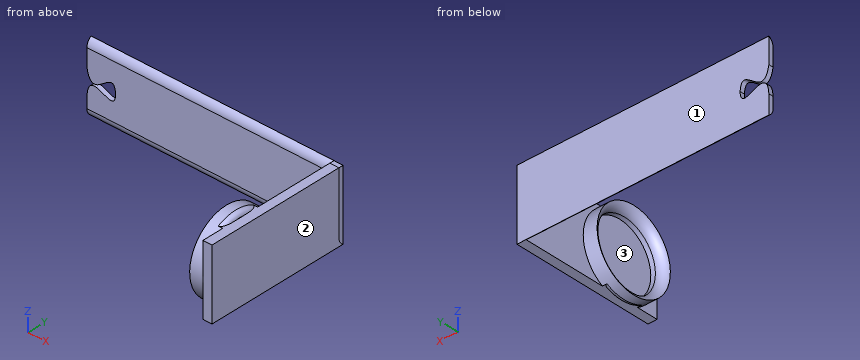
```python
from build123d import *

# Parameters (mm, degrees)
BOSS_EXTRUDE1_DEPTH = 2.54
BOSS_EXTRUDE2_DEPTH = 76.2
SKETCH6_R           = 22
SKETCH6_R_2         = 18.600000000000005
BOSS_EXTRUDE5_DEPTH = 7.660427645478581
FILLET10_R          = 2.5
FILLET11_R          = 2.5
FILLET13_R          = 5.57093307
FILLET15_R          = 5.08
FILLET16_R          = 5.08


with BuildPart() as part:
    # Sketch1 → Boss-Extrude1 (new body)
    with BuildSketch(Plane(origin=(0, 0, 0), x_dir=(1, 0, 0), z_dir=(0, 1, 0))):
        with BuildLine():
            Line((0, 28.293848376378605), (0, 38.694970839027235))
            Line((0, 38.694970839027235), (139, 38.694970839027235))
            Line((139, 38.694970839027235), (139, 0))
            Line((139, 0), (0, 0))
            Line((0, 0), (0, 14.045240588338004))
            add(Edge.make_bspline(
                [(0, 14.045240588338004), (3.0899762489281395, 31.623018189199616), (14.68245796656543, 5.677642965238619), (15.876552294634884, 19.936564793057386)],
                knots=[0, 0, 0, 0, 1, 1, 1, 1], degree=3))
            add(Edge.make_bspline(
                [(0, 28.293848376378605), (1.0033062764081593, 11.15878467888299), (15.658213538640268, 32.998799430672), (15.876552294634884, 19.936564793057386)],
                knots=[0, 0, 0, 0, 1, 1, 1, 1], degree=3))
        make_face()
    extrude(amount=BOSS_EXTRUDE1_DEPTH)

    # Sketch5 → Boss-Extrude2 (add)
    with BuildSketch(Plane.XZ):
        Polygon((138.98190867121684, -38.68428246542061), (133.98190867121684, -38.68428246542061), (133.98190867121684, 0.01068837360662839), (138.98190867121684, 0.010688373606629), align=None)
    extrude(amount=BOSS_EXTRUDE2_DEPTH)

    # Sketch6 → Boss-Extrude5 (add)
    with BuildSketch(Plane.ZY.offset(-133.98190867121684)):
        with Locations(Location((-19.347485419513617, -53.847999999999985, 0), (0, 0, 151.515398593))):
            Circle(SKETCH6_R)
        with Locations((-19.347485419513617, -53.847999999999985)):
            Circle(SKETCH6_R_2, mode=Mode.SUBTRACT)
    extrude(amount=BOSS_EXTRUDE5_DEPTH)

    # Fillet10
    # the kernel refuses this fillet: 2.5 mm, written as the material it takes off along each edge
    with BuildSketch(Plane(origin=(133.98190867121684, -53.847999999999985, -19.347485419513617), x_dir=(0, 0.7041935749471109, -0.7100080344638416), z_dir=(0, 0.7100080344638416, 0.7041935749471109))) as fillet10_piece_1_section:
        with BuildLine():
            CenterArc((22 - FILLET10_R, FILLET10_R), FILLET10_R, 269.9999999999999, 90.00000000000011)
            Line((22 - FILLET10_R, 0), (22, 0))
            Line((22, 0), (22, FILLET10_R))
        make_face()
    fillet10_piece_1 = revolve(axis=Axis((133.98190867121684, -53.847999999999985, -19.347485419513617), (-1, 0, 0)), revolution_arc=89.52886192357941, mode=Mode.PRIVATE)
    fillet10_piece_1 = split(fillet10_piece_1, bisect_by=Plane(origin=(133.27050053527873, -53.847999999999985, -38.68428246542061), z_dir=(0, 0, -1)), keep=Keep.TOP, mode=Mode.PRIVATE)
    add(fillet10_piece_1, mode=Mode.SUBTRACT)

    # Fillet11
    fillet11_edges = [part.edges().sort_by_distance(p)[0] for p in [
        (133.98190867121684, -53.84800000000051, 2.6525145804863826),
    ]]
    fillet(fillet11_edges, radius=FILLET11_R)

    # Fillet13
    # the kernel refuses this fillet: 5.57093307 mm, written as the material it takes off along each edge
    with BuildSketch(Plane(origin=(126.32148102573827, -53.847999999999985, -19.347485419513617), x_dir=(0, 0, 1), z_dir=(0, -1, 0))) as fillet13_piece_1:
        with BuildLine():
            CenterArc((24.170933070445475, -5.130530662517188), FILLET13_R, 112.93516881526322, 67.06483118473678)
            Line((18.600000000000005, -5.130530662517188), (18.488581338591096, -5.130530662517188))
            Line((18.488581338591096, -5.130530662517188), (18.488581338591096, 0))
            Line((18.488581338591096, 0), (18.600000000000005, 0.111418661408905))
            ThreePointArc((18.600000000000005, 0.111418661408905), (20.3, 0.111418661408905), (21.956581338591086, 0.1026106132503628))
            Line((21.956581338591086, 0.1026106132503628), (21.999999999999996, 1.421e-14))
        make_face()
    revolve(axis=Axis((126.32148102573827, -53.847999999999985, -19.347485419513617), (-1, 0, 0)), mode=Mode.SUBTRACT)

    # Fillet15
    # the kernel refuses this fillet: 5.08 mm, written as the material it takes off along each edge
    with BuildSketch(Plane(origin=(-10.998522628063, 0, -38.694970839027235), x_dir=(0, 0, 1), z_dir=(1, 0, 0))) as fillet15_piece_1_section:
        with BuildLine():
            CenterArc((4.3994090512251915, -5.079999999999999), FILLET15_R, 90, 60.00000000000139)
            Line((1.8474e-13, -2.5400000000001057), (0, 0))
            Line((0, 0), (4.3994090512251915, 0))
        make_face()
    fillet15_piece_1 = extrude(amount=160.997045256126, mode=Mode.PRIVATE)
    fillet15_piece_1 = split(fillet15_piece_1, bisect_by=Plane(origin=(133.98190867121684, 0.6664663042665507, -36.831394815078376), z_dir=(-1, 0, 0)), keep=Keep.TOP, mode=Mode.PRIVATE)
    add(fillet15_piece_1, mode=Mode.SUBTRACT)
    with BuildSketch(Plane(origin=(-10.998522628063, 0, -38.694970839027235), x_dir=(0, 0, 1), z_dir=(1, 0, 0))) as fillet15_piece_2_section:
        with BuildLine():
            CenterArc((4.3994090512251915, -5.079999999999999), FILLET15_R, 90, 60.00000000000139)
            Line((1.8474e-13, -2.5400000000001057), (0, 0))
            Line((0, 0), (4.3994090512251915, 0))
        make_face()
    fillet15_piece_2 = extrude(amount=160.997045256126, mode=Mode.PRIVATE)
    fillet15_piece_2 = split(fillet15_piece_2, bisect_by=Plane(origin=(136.48190867121684, 2.530272803909126, -38.68428246542061), z_dir=(0, 0, -1)), keep=Keep.TOP, mode=Mode.PRIVATE)
    add(fillet15_piece_2, mode=Mode.SUBTRACT)
    with BuildSketch(Plane(origin=(-10.998522628063, 0, -38.694970839027235), x_dir=(0, 0, 1), z_dir=(1, 0, 0))) as fillet15_piece_3_section:
        with BuildLine():
            CenterArc((4.3994090512251915, -5.079999999999999), FILLET15_R, 90, 60.00000000000139)
            Line((1.8474e-13, -2.5400000000001057), (0, 0))
            Line((0, 0), (4.3994090512251915, 0))
        make_face()
    fillet15_piece_3 = extrude(amount=160.997045256126, mode=Mode.PRIVATE)
    fillet15_piece_3 = split(fillet15_piece_3, bisect_by=Plane(origin=(138.98190867121684, 0.6664663042665507, -36.831394815078376), z_dir=(1, 0, 0)), keep=Keep.TOP, mode=Mode.PRIVATE)
    add(fillet15_piece_3, mode=Mode.SUBTRACT)

    # Fillet16
    # the kernel refuses this fillet: 5.08 mm, written as the material it takes off along each edge
    with BuildSketch(Plane(origin=(133.98190867121684, 0, 0), x_dir=(0, 0, -1), z_dir=(-1, 0, 0))) as fillet16_piece_1:
        with BuildLine():
            CenterArc((4.399409051225193, -5.079999999999999), FILLET16_R, 90, 60.00000000000139)
            Line((1.8474e-13, -2.5400000000001066), (0, 0))
            Line((0, 0), (4.399409051225193, 0))
        make_face()
    extrude(amount=144.98043129927981, mode=Mode.SUBTRACT)


solid = part.part
```
The model under review builds one solid part; all positions refer to its coordinate system, in mm. Face numbers are marked on the shaded views. Round coordinates to 2 decimals unless told otherwise and drop trailing zeros. Loops run counter-clockwise (first coordinate to the right, second up) from the corner with the lowest first, then second, coordinate; pieces in that order, holes last. Notation, with made-up numbers: M 3,4 L 27,4 A18 ccw 27,24 Z; hole C 22,57.25 d6. An arc over 180 degrees is marked long. Write item = value, one per line.
Item 1: Take a section at B-B on x = 84. Write out the cut boundary in (y, z), then the cut area to 3 significant figures.
Return value:
outline = M 0,-34.3 A5.08 ccw 2.54,-38.69 L 2.54,0 A5.08 ccw 0,-4.4 Z
area = 91.8 mm2
Item 2: For line 1 (Y direction, x = 127.5, z = -3); line 2 (Y direction, x = 133, z = -8); line 3 (X direction, y = -57, z = -21), list the stretches that pass through material, from the lowest coordinate up. Write a range as [from, to].
Return value:
line_1 = [-68.57, -65.79], [-41.91, -39.13], [0.2, 2.54]
line_2 = [-72.7, -68.59], [-39.11, -35], [0, 2.54]
line_3 = [133.98, 138.98]
Item 3: Insertion check: P1, Ø5, axis at y = -52.5, z = -3.5, coming from the +X side; P2, Ø2.5, axis at x = 135.5, y = -26, coming from the +Z side; P3, Ø24, axis at x = 75.5, z = -18, coming from the -Y side. Each pin has a flat end and moves straight along its axis. Give the tip position at first contact, or say it passes through.
Return value:
P1 = 138.98
P2 = 0.01
P3 = 0
Item 4: The part is to be moulded in two halves that separate along Y. For the marked faces 1, 2 and 3, say which applies: released by +Y, released by -Y, zero draft, split by the parting line, or undercut.
Return value:
face_1 = released by +Y
face_2 = zero draft
face_3 = undercut
Item 5: Take a section at A-A on y = -18. Write out the cut boundary in (x, z), then the cut area to 3 significant figures.
Return value:
outline = M 133.98,-38.68 L 138.98,-38.68 L 138.98,0.01 L 133.98,0.01 Z
area = 193 mm2
